Autodesk Inventor part; units mm, degrees
ref_plane "YZ Plane" through (0, 0, 0) normal (1, 0, 0) x (0, 1, 0)
ref_plane "XZ Plane" through (0, 0, 0) normal (0, 1, 0) x (-1, 0, 0)
ref_plane "XY Plane" through (0, 0, 0) normal (0, 0, 1) x (1, 0, 0)
sketch "Sketch1" plane through (0, 0, 0) normal (0, 1, 0) x (-1, 0, 0)
  line L0 (90, 85) -> (-90, 85)
  line L1 (-90, 85) -> (-90, -85)
  line L2 (-90, -85) -> (90, -85)
  line L3 (90, -85) -> (90, 85)
  line L4 (0, -119) -> (0, 119)
  line L5 (-126, 0) -> (126, 0)
  point P0 (0, 0)
  dimension "Length" = 170
  dimension "Width" = 180
extrude "Extrusion1" add sketch "Sketch1" along normal blind 2.5
sketch "Sketch2" plane through (0, 2.5, 0) normal (0, 1, 0) x (1, 0, 0)
  circle A0 centre (-60.5, -74) radius 2.0625
  circle A1 centre (-60.5, -56) radius 2.0625
  circle A2 centre (-35.5, -74) radius 2.0625
  circle A3 centre (-35.5, -56) radius 2.0625
  line L0 (-60.5, -74) -> (-60.5, -56) construction
  line L1 (-60.5, -56) -> (-35.5, -56) construction
  line L2 (-35.5, -56) -> (-35.5, -74) construction
  line L3 (-35.5, -74) -> (-60.5, -74) construction
  line L4 (-90, 85) -> (-90, -85) construction
  line L5 (-90, -85) -> (90, -85) construction
  circle A4 centre (-80, -65) radius 2.0625
  point P0 (0, 0)
  dimension "d4" = 4.125
  dimension "d5" = 18
  dimension "d6" = 25
  dimension "d7" = 29.5
  dimension "d8" = 11
  dimension "d9" = 4.125
  dimension "d10" = 10
  dimension "d11" = 20
extrude "Extrusion2" cut sketch "Sketch2" against normal up to next
mirror "Mirror1" about plane through (0, 0, 0) normal (0, 0, 1) of "Extrusion2"
mirror "Mirror2" about plane through (0, 0, 0) normal (1, 0, 0) of "Extrusion2", "Mirror1"
sketch "Sketch3" plane through (0, 2.5, 0) normal (0, 1, 0) x (1, 0, 0)
  circle A0 centre (-37.5, -15) radius 2.0625
  circle A1 centre (-37.5, 15) radius 2.0625
  circle A2 centre (-22.5, -15) radius 2.0625
  circle A3 centre (-22.5, 15) radius 2.0625
  line L0 (-22.5, 15) -> (-37.5, 15) construction
  line L1 (-37.5, 15) -> (-37.5, -15) construction
  line L2 (-37.5, -15) -> (-22.5, -15) construction
  line L3 (-22.5, -15) -> (-22.5, 15) construction
  line L4 (-22.5, 15) -> (-37.5, -15) construction
  line L5 (-37.5, 15) -> (-22.5, -15) construction
  line L6 (-90, 85) -> (-90, -85) construction
  line L7 (144.445, 0) -> (-144.445, 0) construction
  point P0 (0, 0)
  point P1 (-30, 0)
  point P2 (-30, 0)
  dimension "d14" = 30
  dimension "d15" = 4.125
  dimension "d16" = 15
  dimension "d17" = 60
extrude "Extrusion3" cut sketch "Sketch3" against normal up to next
properties part number "Base Plate" material "Aluminum 6061"
Input: part model. Units: mm. Frame: model coordinates. Give positions to 0.01 mm unless a question says otherwise; leave off trailing zeros. Order: outer loops, then holes, each group sorted by start corner. A loop starts at its lowest first (then second) coordinate and runs counter-clockwise, first axis right, second up. Notation, with made-up numbers: (26.25, 85.5) - (43.25, 85.5) arc R10 cw to (43.25, 95.5) - close; hole circle Ø8 at (30.25, 39.25). An arc over 180 degrees is marked (long way). Use a Markdown table: item, result.
(1) Section query B-B (x = -60.5). Output: boundary loops of the cut face in (y, z), then the cut area to 3 significant figures.
Computed values:
| item | result |
|---|---|
| outline | (0, -85) - (2.5, -85) - (2.5, -76.06) - (0, -76.06) - close; (0, -71.94) - (2.5, -71.94) - (2.5, -58.06) - (0, -58.06) - close; (0, -53.94) - (2.5, -53.94) - (2.5, 53.94) - (0, 53.94) - close; (0, 58.06) - (2.5, 58.06) - (2.5, 71.94) - (0, 71.94) - close; (0, 76.06) - (2.5, 76.06) - (2.5, 85) - (0, 85) - close |
| area | 384 mm2 |
(2) Section query A-A (z = -56). Output: boundary loops of the cut face in (x, y).
Computed values:
| item | result |
|---|---|
| outline | (-90, 0) - (-62.56, 0) - (-62.56, 2.5) - (-90, 2.5) - close; (-58.44, 0) - (-37.56, 0) - (-37.56, 2.5) - (-58.44, 2.5) - close; (-33.44, 0) - (33.44, 0) - (33.44, 2.5) - (-33.44, 2.5) - close; (37.56, 0) - (58.44, 0) - (58.44, 2.5) - (37.56, 2.5) - close; (62.56, 0) - (90, 0) - (90, 2.5) - (62.56, 2.5) - close |
(3) Section query C-C (z = 15). Output: boundary loops of the cut face in (x, y), then the cut area to 3 significant figures.
Computed values:
| item | result |
|---|---|
| outline | (-90, 0) - (-39.56, 0) - (-39.56, 2.5) - (-90, 2.5) - close; (-35.44, 0) - (-24.56, 0) - (-24.56, 2.5) - (-35.44, 2.5) - close; (-20.44, 0) - (90, 0) - (90, 2.5) - (-20.44, 2.5) - close |
| area | 429 mm2 |
(4) Line query: line 1 (X direction, y = 1.75, z = -15); line 2 (Z direction, x = 60.5, y = 1.6); line 3 (Z direction, x = -22.5, y = 1.3). Output: solid intervals per line, ascending. Write a range as from..to.
Computed values:
| item | result |
|---|---|
| line 1 | x = -90..-39.56, -35.44..-24.56, -20.44..90 |
| line 2 | z = -85..-76.06, -71.94..-58.06, -53.94..53.94, 58.06..71.94, 76.06..85 |
| line 3 | z = -85..-17.06, -12.94..12.94, 17.06..85 |
(5) Draft query along X for faces 1 (the flat face through (1, 0, 1)), 2 (the cylindrical face through (58.533, 1.268, -73.38)). Return one class per face: released by +X, released by -X, zero draft, split by the parting line, or undercut.
Computed values:
| item | result |
|---|---|
| face 1 | zero draft |
| face 2 | undercut |
(6) Section query D-D (x = -80). Output: boundary loops of the cut face in (y, z), then the cut area to 3 significant figures.
Computed values:
| item | result |
|---|---|
| outline | (0, -85) - (2.5, -85) - (2.5, -67.06) - (0, -67.06) - close; (0, -62.94) - (2.5, -62.94) - (2.5, 62.94) - (0, 62.94) - close; (0, 67.06) - (2.5, 67.06) - (2.5, 85) - (0, 85) - close |
| area | 404 mm2 |
